Geometry: final body of the model. Coordinates: model frame, mm. A direction names the side the tool comes from. Give positions to 0.01 mm unless a question says otherwise; leave off trailing zeros. Loops run counter-clockwise (first coordinate to the right, second up) from the corner with the lowest first, then second, coordinate; pieces in that order, holes last. Notation, with made-up numbers: (65, -7) -> (82, -7) arc R23 cw to (82, 32) -> close; hole circle Ø11 at (26.25, 73.5). An arc over 180 degrees is marked (long way). Answer in a Markdown table with one row per item. Add a question column.
1) Section query B-B (y = -1.7). Return the cut outline in (x, z), plus the area to 3 significant figures.
2) Section query C-C (z = 2.75). Return the cut outline in (x, y).
3) Section query A-A (x = -4.5). Return the cut outline in (y, z), plus the area to 3 significant figures.
4) Access query for faces 1 (the flat face through (-0.5, -2.5, 0)), 2 (the flat face through (-11.5, -2.5, 0)). Directions: +Z, -Z, +X, -X, +Y, -Y. A direction counts if a zero-diameter tool reaches every point of the face in a straight line with its end or side. Return the directions, or none.
5) Line query: line 1 (Y direction, x = -6, z = 6.25); line 2 (X direction, y = -2.45, z = 5.75); line 3 (Z direction, x = -9.5, y = -4.8). Output: solid intervals per line, ascending. Write a range as from..to.
6) Draft query along Y for faces 3 (the cylindrical face through (-6.478, -0.322, 3.902)), 4 (the flat face through (0, -2, 5)), 5 (the flat face through (-6, -5, 5)). Return one class per face: +Y half, -Y half, draft (parallel to the pull), parting line (faces both ways), or undercut.
7) First-contact query: P1, Ø1.1, axis at x = -0.5, y = -2.5, coming from the -Z side; P2, Ø0.5, axis at y = -3.5, z = -0.5, coming from the +X side; P3, Ø1, axis at x = -7, y = -3, coming from the -Z side; P4, Ø0.8, axis at y = -3.5, z = -0.5, coming from the -X side. Flat tips, straight axial feed; report the tip coordinate or a pass-through.
```python
from build123d import *

# Parameters (mm, degrees)
F1_DEPTH = 5
F3_DEPTH = 2
F4_R     = 2.20671025
F5_DEPTH = 25


with BuildPart() as f1:
    # F0 (on Front) → F1 (new body)
    with BuildSketch(Plane.XZ):
        Polygon((0, 11), (-12, 11), (-12, 0), (-11, 0), (-11, -1), (-1, -1), (-1, 0), (0, 0), align=None)
    extrude(amount=F1_DEPTH)

    # F2 (on face) → F3 (join)
    with BuildSketch(Plane(origin=(0, 0, -1), x_dir=(1, 0, 0), z_dir=(0, 0, -1))):
        with BuildLine():
            ThreePointArc((-5.6578661307, 0), (-4.1151479271, 0.8341224011), (-3.5, 2.4764782283))
            ThreePointArc((-3.5, 2.4764782283), (-7.6423558273, 4.3613303012), (-6.3421338693, 0))
            Line((-6.3421338693, 0), (-5.6578661307, 0))
        make_face()
    extrude(amount=F3_DEPTH)

    # F4 (on face) → F5 (cut)
    with BuildSketch(Plane(origin=(0, 0, -3), x_dir=(1, 0, 0), z_dir=(0, 0, -1))):
        with Locations((-6, 2.4764782283)):
            Circle(F4_R)
    extrude(amount=-F5_DEPTH, mode=Mode.SUBTRACT)


solid = f1.part
```
Evaluation:
| question | item | result |
|---|---|---|
| 1 | outline | (-12, 0) -> (-11, 0) -> (-11, -1) -> (-8.38, -1) -> (-8.38, -3) -> (-8.07, -3) -> (-8.07, 11) -> (-12, 11) -> close; (-3.93, -3) -> (-3.62, -3) -> (-3.62, -1) -> (-1, -1) -> (-1, 0) -> (0, 0) -> (0, 11) -> (-3.93, 11) -> close |
| 1 | area | 93.7 mm² |
| 2 | outline | (-12, -5) -> (0, -5) -> (0, 0) -> (-12, 0) -> close; hole circle Ø4.41 at (-6, -2.48) |
| 3 | outline | (-5, -1) -> (-4.48, -1) -> (-4.48, -3) -> (-4.09, -3) -> (-4.09, 11) -> (-5, 11) -> close; (-0.86, -3) -> (-0.48, -3) -> (-0.48, -1) -> (0, -1) -> (0, 11) -> (-0.86, 11) -> close |
| 3 | area | 22.7 mm² |
| 4 | face 1 | -Z, +X, +Y, -Y |
| 4 | face 2 | -Z, -X, +Y, -Y |
| 5 | line 1 | -5..-4.68, -0.27..0 |
| 5 | line 2 | -12..-8.21, -3.79..0 |
| 5 | line 3 | -1..11 |
| 6 | face 3 | undercut |
| 6 | face 4 | draft |
| 6 | face 5 | -Y half |
| 7 | P1 | z = -1 |
| 7 | P2 | x = -1 |
| 7 | P3 | through |
| 7 | P4 | x = -11 |
